For this review, use the dimensioned drawing (mm, ordinates from the lowest corner) and the shaded views. A direction names the side the tool comes from. Round coordinates to 2 decimals unless told otherwise and drop trailing zeros. Write each loop counter-clockwise with the first axis right and the second up, starting at its lowest first coordinate (ties: lowest second). Pieces come first, ordered by that corner, then holes.
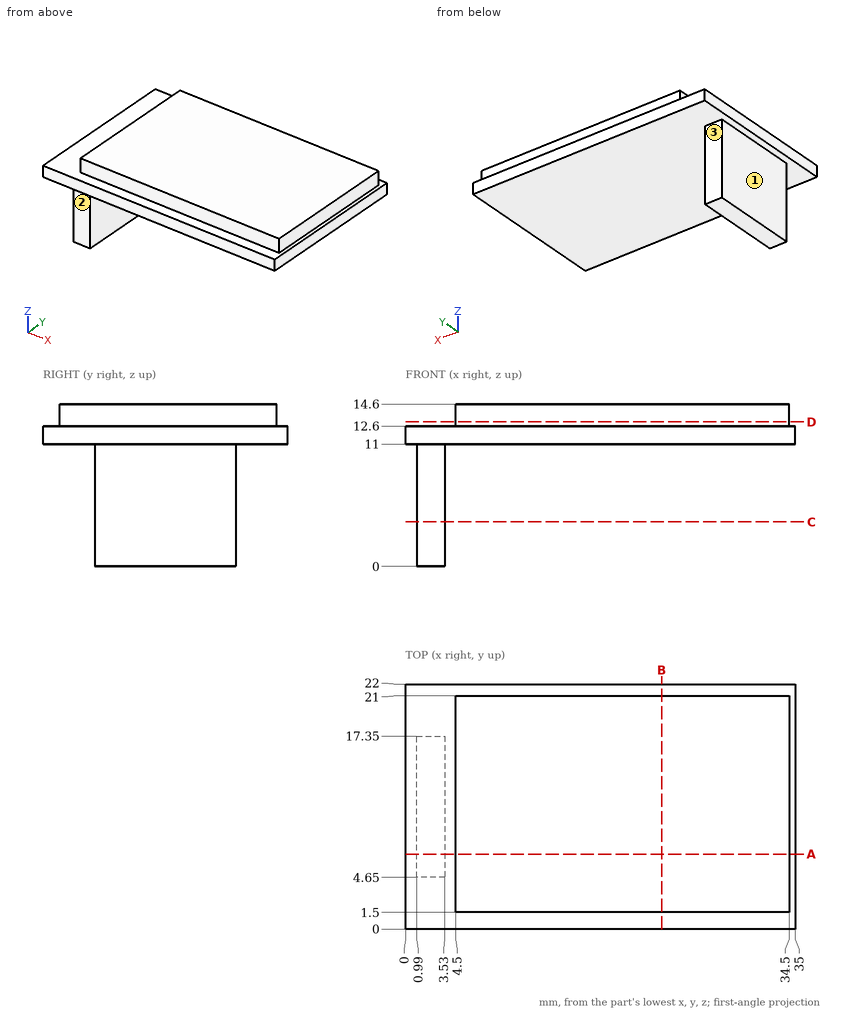
(1) We need section B-B, the plane x = 23. Give the boundary of the cut face in (y, z), and give its area (3 significant figures).
Geometry check:
outline: (0, 11) - (22, 11) - (22, 12.6) - (21, 12.6) - (21, 14.6) - (1.5, 14.6) - (1.5, 12.6) - (0, 12.6) - close
area: 74.2 mm2
(2) For the marked faces 1, 2 and 3, list the 3-axis set-ups (+Z, -Z, +X, -X, +Y, -Y) from which the entire face can be reached by the end or side of a thin tool; tool diameter is ignored.
Geometry check:
face 1: -Z, -X, +Y, -Y
face 2: -Z, +X, -X, -Y
face 3: -Z, +X, -X, +Y
(3) We need section C-C, the plane z = 4. Give the boundary of the cut face in (x, y).
Geometry check:
outline: (0.99, 4.65) - (3.53, 4.65) - (3.53, 17.35) - (0.99, 17.35) - close
(4) We need section D-D, the plane z = 13. Give the boundary of the cut face in (x, y), and give its area (3 significant figures).
Geometry check:
outline: (4.5, 1.5) - (34.5, 1.5) - (34.5, 21) - (4.5, 21) - close
area: 585 mm2
(5) For pin 1 Ø5.5 at (y, z) = (13, 6) entering from +X; pin 2 Ø0.8 at (x, z) = (1.5, 5.5) entering from -Y; pin 3 Ø6 at (x, y) = (29.5, 2.5) entering from -Z, all flat-tipped, find the tip position at first contact; note any pin that passes through.
Geometry check:
pin 1: stops at x = 3.53
pin 2: stops at y = 4.65
pin 3: stops at z = 11
(6) For line 1 along Z through (x, y) = (32, 5); line 2 along X through (y, z) = (12.75, 10); line 3 along Z through (x, y) = (4, 1.25), list the stretches that pass through material, from the lowest coordinate up.
Geometry check:
line 1: z = 11 to 14.6
line 2: x = 0.99 to 3.53
line 3: z = 11 to 12.6
(7) We need section A-A, the plane y = 6.75. Give the boundary of the cut face in (x, z), and give its area (3 significant figures).
Geometry check:
outline: (0, 11) - (0.99, 11) - (0.99, 0) - (3.53, 0) - (3.53, 11) - (35, 11) - (35, 12.6) - (34.5, 12.6) - (34.5, 14.6) - (4.5, 14.6) - (4.5, 12.6) - (0, 12.6) - close
area: 144 mm2
